Read the model definition and answer for the solid it produces. Units are mm, in the model's axes. Face numbers are marked on the shaded views. Coordinates: 2 decimals unless noted, no trailing zeros. Loops run counter-clockwise (first coordinate to the right, second up) from the corner with the lowest first, then second, coordinate; pieces in that order, holes last. Notation, with made-up numbers: (-1.75, -7.75) -> (37.25, -7.75) arc R16 cw to (37.25, 5.25) -> close; hole circle Ø6 at (-36, 89). An arc over 180 degrees is marked (long way). Answer in a Markdown table with one row per item.
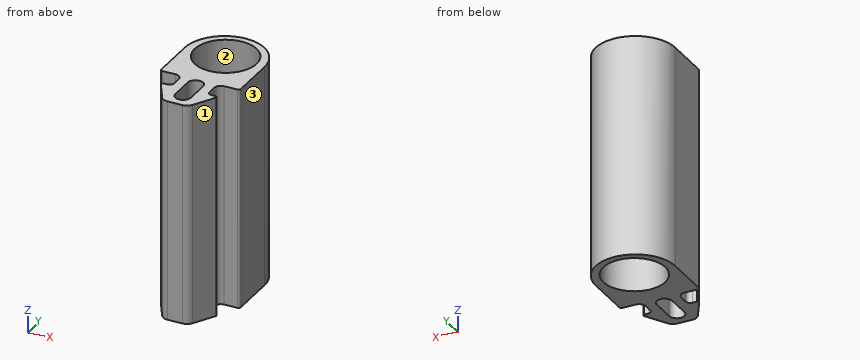
```python
from build123d import *

# Parameters (mm, degrees)
ESQUISSE1_R        = 7
BOSS_EXTRU_1_DEPTH = 50


with BuildPart() as part:
    # Esquisse1 → Boss.-Extru.1 (new body)
    with BuildSketch(Plane.XY.offset(20)):
        with BuildLine():
            Line((-9, 10.864586864), (-9, 0.523924837))
            ThreePointArc((-9, 0.523924837), (-8.854824532, 0.14661401), (-8.478070356, 0))
            Line((-8.478070356, 0), (-5.5, 0))
            ThreePointArc((-5.5, 0), (-4.439339828, -0.439339828), (-4, -1.5))
            Line((-4, -1.5), (-4, -3.5))
            ThreePointArc((-4, -3.5), (-4.292893219, -4.207106781), (-5, -4.5))
            Line((-5, -4.5), (-6.016007613, -4.5))
            ThreePointArc((-6.016007613, -4.5), (-6.227713349, -4.802430523), (-6.174193657, -5.16769643))
            Line((-6.174193657, -5.16769643), (-3.440043573, -9.90338329))
            ThreePointArc((-3.440043573, -9.90338329), (-2.707992766, -10.635434098), (-1.707992766, -10.90338329))
            Line((-1.707992766, -10.90338329), (1.707992766, -10.90338329))
            ThreePointArc((1.707992766, -10.90338329), (2.707992766, -10.635434098), (3.440043573, -9.90338329))
            Line((3.440043573, -9.90338329), (6.174193657, -5.16769643))
            ThreePointArc((6.174193657, -5.16769643), (6.227713349, -4.802430523), (6.016007614, -4.5))
            Line((6.016007614, -4.5), (5, -4.5))
            ThreePointArc((5, -4.5), (4.292893219, -4.207106781), (4, -3.5))
            Line((4, -3.5), (4, -1.5))
            ThreePointArc((4, -1.5), (4.439339828, -0.439339828), (5.5, 0))
            Line((5.5, 0), (8.478070356, 0))
            ThreePointArc((8.478070356, 0), (8.854824532, 0.14661401), (9, 0.523924837))
            Line((9, 0.523924837), (9, 10.864586864))
            ThreePointArc((9, 10.864586864), (0, 19.864586864), (-9, 10.864586864))
        make_face()
        with Locations((0, 11.36)):
            Circle(ESQUISSE1_R, mode=Mode.SUBTRACT)
        with BuildLine():
            Line((1.75, -1.95338329), (1.75, -7.351528839))
            ThreePointArc((1.75, -7.351528839), (0, -9.101528839), (-1.75, -7.351528839))
            Line((-1.75, -7.351528839), (-1.75, -1.95338329))
            ThreePointArc((-1.75, -1.95338329), (0, -0.20338329), (1.75, -1.95338329))
        make_face(mode=Mode.SUBTRACT)
    extrude(amount=-BOSS_EXTRU_1_DEPTH)


solid = part.part
```
1. A cutting plane is placed at D-D on x = 0. Give the vertices of the cut face in (y, z).
A:
| item | result |
|---|---|
| outline | (-10.9, -30) -> (-9.1, -30) -> (-9.1, 20) -> (-10.9, 20) -> close; (-0.2, -30) -> (4.36, -30) -> (4.36, 20) -> (-0.2, 20) -> close; (18.36, -30) -> (19.86, -30) -> (19.86, 20) -> (18.36, 20) -> close |
2. The mould has two halves that part along Y. Classify the marked faces 1, 2 and 3: pulls with the +Y half, pulls with the -Y half, needs draft (parallel to the pull), parting line crosses it, or undercut.
A:
| item | result |
|---|---|
| face 1 | pulls with the -Y half |
| face 2 | undercut |
| face 3 | needs draft |
3. A cutting plane is placed at A-A on z = -18. Give the vertices of the cut face in (x, y), and give its area (3 significant figures).
A:
| item | result |
|---|---|
| outline | (-9, 0.52) arc R0.5 ccw to (-8.48, 0) -> (-5.5, 0) arc R1.5 cw to (-4, -1.5) -> (-4, -3.5) arc R1 cw to (-5, -4.5) -> (-6.02, -4.5) arc R0.5 ccw to (-6.17, -5.17) -> (-3.44, -9.9) arc R2 ccw to (-1.71, -10.9) -> (1.71, -10.9) arc R2 ccw to (3.44, -9.9) -> (6.17, -5.17) arc R0.5 ccw to (6.02, -4.5) -> (5, -4.5) arc R1 cw to (4, -3.5) -> (4, -1.5) arc R1.5 cw to (5.5, 0) -> (8.48, 0) arc R0.5 ccw to (9, 0.52) -> (9, 10.86) arc R9 ccw to (-9, 10.86) -> close; hole circle Ø14 at (0, 11.36); hole (-1.75, -7.35) arc R1.75 ccw to (1.75, -7.35) -> (1.75, -1.95) arc R1.75 ccw to (-1.75, -1.95) -> close |
| area | 237 mm2 |
4. Given pin 1 Ø0.5 at (x, z) = (5.5, 6.5) entering from +Y; pin 2 Ø0.9 at (x, z) = (-6.5, -9) entering from -Y; pin 3 Ø4.5 at (y, z) = (-4.5, 5) entering from +X, each flat-ended and moving along its own axis, determine where each tip first touches the part or whether it passes through.
A:
| item | result |
|---|---|
| pin 1 | stops at y = 18.17 |
| pin 2 | stops at y = -5.38 |
| pin 3 | stops at x = 6.24 |
5. Find the intervals of material crossed by probe 1 along Y at (x, z) = (0, -19.5); probe 2 along X at (y, z) = (11, -1.5); probe 3 along Y at (x, z) = (3.25, -6.5), in increasing order.
A:
| item | result |
|---|---|
| probe 1 | y = -10.9 to -9.1, -0.2 to 4.36, 18.36 to 19.86 |
| probe 2 | x = -9 to -6.99, 6.99 to 9 |
| probe 3 | y = -10.18 to 5.16, 17.56 to 19.26 |
6. A cutting plane is placed at C-C on x = 2.5. Give the vertices of the cut face in (y, z).
A:
| item | result |
|---|---|
| outline | (-10.74, -30) -> (4.82, -30) -> (4.82, 20) -> (-10.74, 20) -> close; (17.9, -30) -> (19.51, -30) -> (19.51, 20) -> (17.9, 20) -> close |
7. A cutting plane is placed at B-B on y = 11.36. Give the vertices of the cut face in (x, z), and give its area (3 significant figures).
A:
| item | result |
|---|---|
| outline | (-8.99, -30) -> (-7, -30) -> (-7, 20) -> (-8.99, 20) -> close; (7, -30) -> (8.99, -30) -> (8.99, 20) -> (7, 20) -> close |
| area | 199 mm2 |
